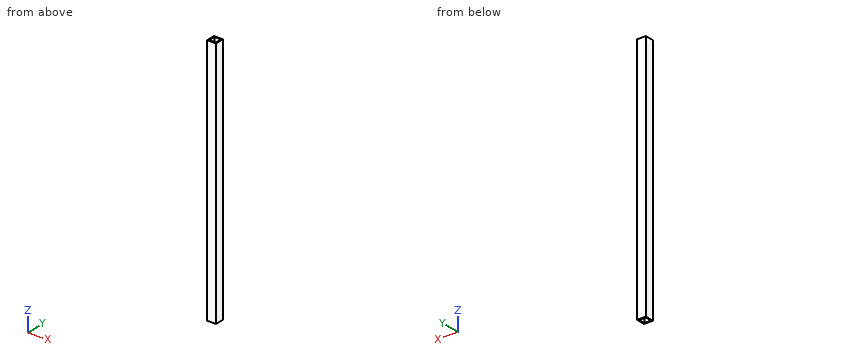
Autodesk Inventor part; units mm, degrees
ref_plane "Start Plane" through (0, 0, 19.05) normal (0, 0, 1) x (1, 0, 0)
ref_plane "End Plane" through (0, 0, 742.95) normal (0, 0, 1) x (1, 0, 0)
ref_plane "Work Plane5" through (19.05, 76.2, 742.95) normal (0, 0, 1) x (1, 0, 0)
ref_plane "Start Plane" through (0, 0, 19.05) normal (0, 0, 1) x (1, 0, 0)
ref_plane "End Plane" through (0, 0, 742.95) normal (0, 0, 1) x (1, 0, 0)
sketch "Sketch" plane through (0, 0, 0) normal (0, 0, 1) x (1, 0, 0)
  line L0 (-12.7, 12.7) -> (12.7, 12.7)
  line L1 (12.7, 12.7) -> (12.7, -12.7)
  line L2 (12.7, -12.7) -> (-12.7, -12.7)
  line L3 (-12.7, -12.7) -> (-12.7, 12.7)
  line L4 (9.525, 9.525) -> (-9.525, 9.525)
  line L5 (-9.525, 9.525) -> (-9.525, -9.525)
  line L6 (-9.525, -9.525) -> (9.525, -9.525)
  line L7 (9.525, -9.525) -> (9.525, 9.525)
  point P0 (0, 0)
  point P1 (0, 12.7)
  point P2 (-12.7, 0)
  dimension "width" = 25.4
  dimension "d1" = 3.175
extrude "Body" add sketch "Sketch" along normal up to surface (723.9 mm away) from surface at 19.05
sketch "Sketch4" plane through (0, 0, 0) normal (0, 0, 1) x (1, 0, 0)
  line L0 (0, 0) -> (10, 0)
ref_plane "Work Plane4" through (0, 0, 0) normal (0, -1, 0) x (1, 0, 0)
sketch "Sketch5" plane through (0, 0, 0) normal (0, -1, 0) x (1, 0, 0)
  line L0 (-2, 19.05) -> (12, 19.05)
  line L1 (-2, 742.95) -> (12, 742.95)
  dimension "d9" = 723.9
ref_plane "Work Plane5" through (19.05, 76.2, 742.95) normal (0, 0, 1) x (1, 0, 0)
split "Split1" plane through (19.05, 76.2, 742.95) removes the side toward (0, 0, 1)
ref_plane "Work Plane6" through (-19.05, 76.2, 19.05) normal (0, 0, -1) x (-1, 0, 0)
split "Split2" plane through (-19.05, 76.2, 19.05) removes the side toward (0, 0, -1)
equation "\"G_OFFSET_START\" = -19.05"
equation "\"G_OFFSET_END\" = -19.05"
equation "\"d4\" = -G_OFFSET_START"
equation "\"d5\" = length + G_OFFSET_END"
equation "\"G_L\" = 762"
properties part number "Square Tube Profile" material "Aluminum-6061"
Build history of the part. All positions in model axes, mm. Coordinates: 2 decimals unless noted, no trailing zeros. Order: outer loops, then holes, each group sorted by start corner. A loop starts at its lowest first (then second) coordinate and runs counter-clockwise, first axis right, second up.
Item 1: Drill centre line: L1, parallel to Y at x = -0.25, z = 622 (3 decimals). Where is it in solid material? Low to high.
Filled in:
L1: y = -12.7 to -9.525, 9.525 to 12.7
Item 2: Saw through at A-A on x = 2.5. List the corners of the cut face in (y, z) (3 decimals).
Filled in:
outline: (-12.7, 19.05) - (-9.525, 19.05) - (-9.525, 742.95) - (-12.7, 742.95) - close; (9.525, 19.05) - (12.7, 19.05) - (12.7, 742.95) - (9.525, 742.95) - close
Item 3: Drop a flat-ended pin along its axis: pin 1 Ø2 at (x, y) = (3.5, 9.5) entering from -Z. Give the stop position or say it passes through.
Filled in:
pin 1: stops at z = 19.05
Item 4: Saw through at B-B on z = 219.5. List the corners of the cut face in (x, y) (3 decimals), then the cut area to 3 significant figures.
Filled in:
outline: (-12.7, -12.7) - (12.7, -12.7) - (12.7, 12.7) - (-12.7, 12.7) - close; hole (-9.525, -9.525) - (9.525, -9.525) - (9.525, 9.525) - (-9.525, 9.525) - close
area: 282 mm2
